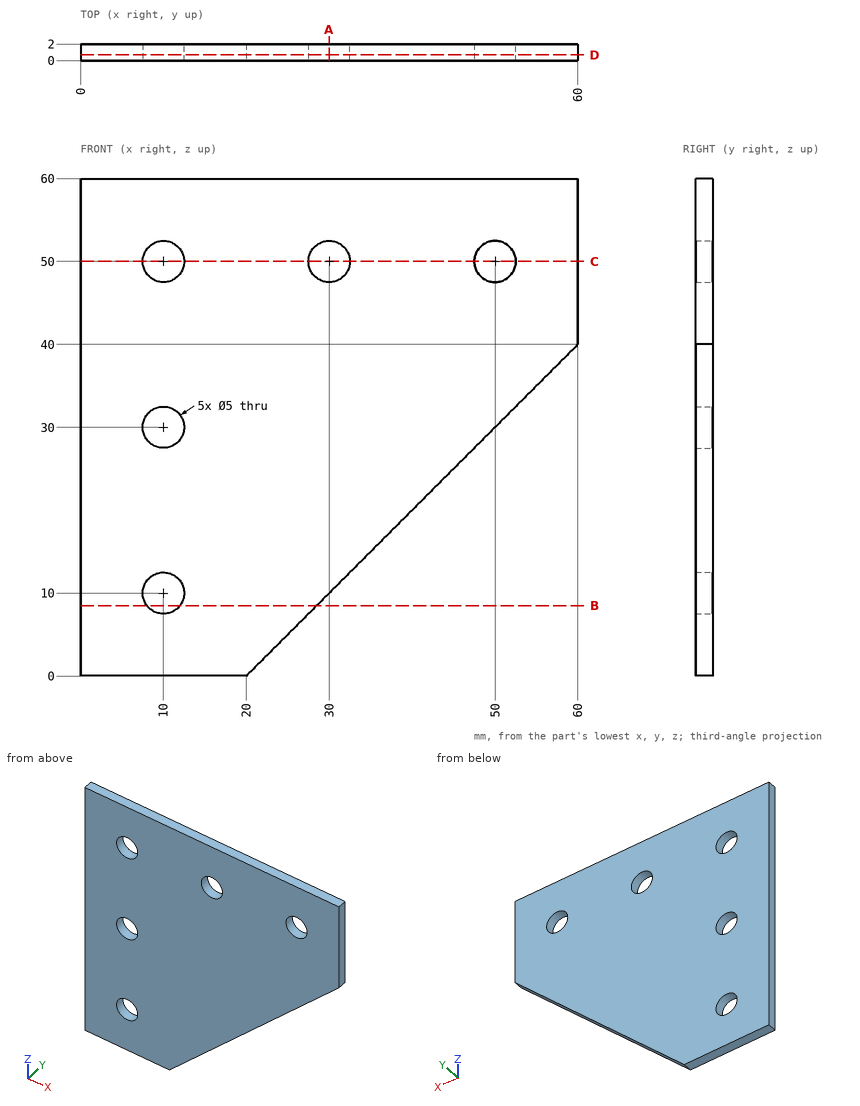
Geometry: see drawing. Coordinates: mm, zero at the bounding-box minimum. Give positions to 0.01 mm unless a question says otherwise; leave off trailing zeros. Loops run counter-clockwise (first coordinate to the right, second up) from the corner with the lowest first, then second, coordinate; pieces in that order, holes last. Notation, with made-up numbers: M 42.25,26 L 60.25,26 A31 cw 60.25,59 Z; hole C 17,31 d8. An arc over 180 degrees is marked long. Answer as CSV lines item,"result". Start each with the question number.
1. Section C-C on z = 50. Return loops of the section in (x, y).
2. Line query: L1, parallel to Z at x = 10, y = 0.8; L2, parallel to X at y = 0.1, z = 28; L3, parallel to Z at x = 52, y = 0.9. Output: solid intervals per line, ascending.
3. Section B-B on z = 8.5. Return loops of the section in (x, y).
4. Section D-D on y = 0.7. Return loops of the section in (x, z), plus the area to 3 significant figures.
5. Section A-A on x = 30. Return loops of the section in (y, z).
Computed values:
1,outline,"M 0,0 L 7.5,0 L 7.5,2 L 0,2 Z; M 12.5,0 L 27.5,0 L 27.5,2 L 12.5,2 Z; M 32.5,0 L 47.5,0 L 47.5,2 L 32.5,2 Z; M 52.5,0 L 60,0 L 60,2 L 52.5,2 Z"
2,L1,"z = 0 to 7.5, 12.5 to 27.5, 32.5 to 47.5, 52.5 to 60"
2,L2,"x = 0 to 8.5, 11.5 to 48"
2,L3,"z = 32 to 48.5, 51.5 to 60"
3,outline,"M 0,0 L 8,0 L 8,2 L 0,2 Z; M 12,0 L 28.5,0 L 28.5,2 L 12,2 Z"
4,outline,"M 0,0 L 20,0 L 60,40 L 60,60 L 0,60 Z; hole C 10,10 d5; hole C 10,30 d5; hole C 10,50 d5; hole C 30,50 d5; hole C 50,50 d5"
4,area,"2,700 mm²"
5,outline,"M 0,10 L 2,10 L 2,47.5 L 0,47.5 Z; M 0,52.5 L 2,52.5 L 2,60 L 0,60 Z"
